Autodesk Inventor part; units mm, degrees
ref_plane "YZ Plane" through (0, 0, 0) normal (1, 0, 0) x (0, 1, 0)
ref_plane "XZ Plane" through (0, 0, 0) normal (0, 1, 0) x (-1, 0, 0)
ref_plane "XY Plane" through (0, 0, 0) normal (0, 0, 1) x (1, 0, 0)
sketch "Sketch1" plane through (0, 0, 0) normal (0, 1, 0) x (-1, 0, 0)
  line L0 (0, 0) -> (-228.6, 0)
  line L1 (-228.6, 0) -> (-228.6, -25.4)
  line L2 (-228.6, -25.4) -> (0, -25.4)
  line L3 (0, -25.4) -> (0, 0)
  dimension "d0" = 228.6
  dimension "d1" = 25.4
extrude "Extrusion1" add sketch "Sketch1" along normal blind 11.938
sketch "Sketch4" plane through (0, 11.938, 0) normal (0, 1, 0) x (1, 0, 0)
  line L0 (228.6, 25.4) -> (0, 25.4)
  line L1 (114.3, 25.4) -> (114.3, 0) construction
  line L2 (0, 0) -> (228.6, 0)
  circle A0 centre (114.3, 12.7) radius 2.3812
  line L3 (0, 25.4) -> (0, 0)
  line L4 (0, 12.7) -> (12.7, 12.7)
  line L5 (0, 12.7) -> (12.7, 12.7) construction
  circle A1 centre (12.7, 12.7) radius 2.3812
  dimension "d40" = 12.7
  dimension "d42" = 4.7625
hole "Hole3" at (114.3, 11.938, -12.7) at (12.7, 11.938, -12.7) direction (0, -1, 0) diameter 4.7625 end through all
properties part number "track"
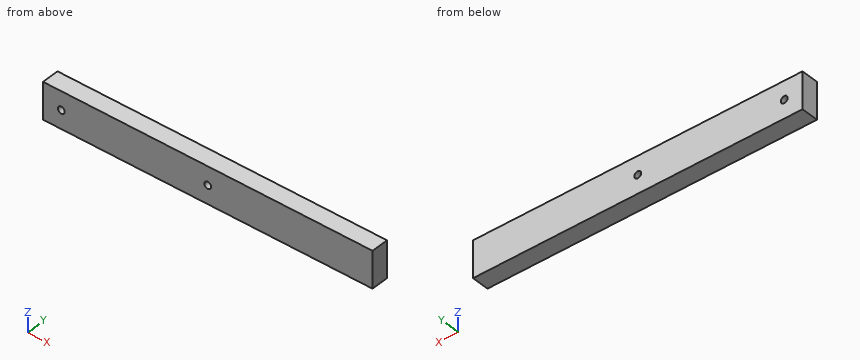
The model under review builds one solid part; all positions refer to its coordinate system, in mm. Round coordinates to 2 decimals unless told otherwise and drop trailing zeros. Order: outer loops, then holes, each group sorted by start corner. A loop starts at its lowest first (then second) coordinate and runs counter-clockwise, first axis right, second up. Notation, with made-up numbers: (17, 50.5) - (35, 50.5) arc R25 ccw to (35, 68.5) - close; hole circle Ø6 at (-33, 88.25). An arc over 180 degrees is marked (long way). Answer in a Markdown table with one row per item.
(1) Take a section at B-B on x = 12.7. Write out the cut boundary in (y, z).
Result set:
| item | result |
|---|---|
| outline | (0, -25.4) - (11.94, -25.4) - (11.94, -15.08) - (0, -15.08) - close; (0, -10.32) - (11.94, -10.32) - (11.94, 0) - (0, 0) - close |
(2) For line 1 (X direction, y = 3, z = -12.7); line 2 (Z direction, x = 114.3, y = 4.5); line 3 (X direction, y = 9, z = -14.75), list the stretches that pass through material, from the lowest coordinate up. Write a range as from..to.
Result set:
| item | result |
|---|---|
| line 1 | x = 0..10.32, 15.08..111.92, 116.68..228.6 |
| line 2 | z = -25.4..-15.08, -10.32..0 |
| line 3 | x = 0..11.49, 13.91..113.09, 115.51..228.6 |
(3) Take a section at A-A on z = -12.7. Write out the cut boundary in (x, y).
Result set:
| item | result |
|---|---|
| outline | (0, 0) - (10.32, 0) - (10.32, 11.94) - (0, 11.94) - close; (15.08, 0) - (111.92, 0) - (111.92, 11.94) - (15.08, 11.94) - close; (116.68, 0) - (228.6, 0) - (228.6, 11.94) - (116.68, 11.94) - close |
